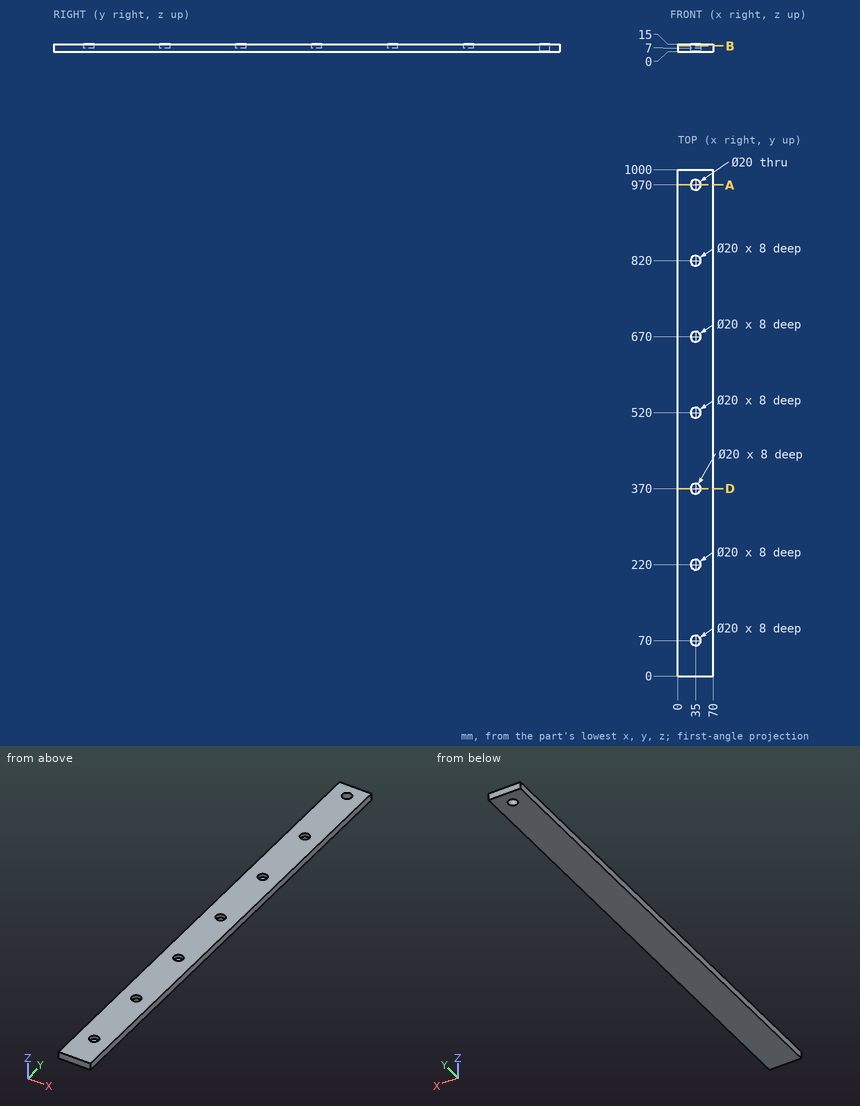
Answer from the drawing. Dimensions are ordinates in mm from the lowest x, y and z of the part. Coordinates: 2 decimals unless noted, no trailing zeros. Loops run counter-clockwise (first coordinate to the right, second up) from the corner with the lowest first, then second, coordinate; pieces in that order, holes last.
1) Consider probe 1 along X at (y, z) = (520, 9.75); probe 2 along Y at (x, z) = (27.5, 5); probe 3 along Y at (x, z) = (43, 4.75). Determine where each line is inside the solid, lowest interval first.
Results:
probe 1: x = 0 to 25, 45 to 70
probe 2: y = 0 to 963.39, 976.61 to 1000
probe 3: y = 0 to 964, 976 to 1000
2) Section A-A (y = 970) is taken. Give the vertices of the cut face in (x, z), plus the area to 3 significant figures.
Results:
outline: (0, 0) - (25, 0) - (25, 15) - (0, 15) - close; (45, 0) - (70, 0) - (70, 15) - (45, 15) - close
area: 750 mm2
3) Flat-ended cylindrical pins translate along their axes: pin 1 (12 mm diameter, centred on x = 35, y = 220, fed in from -Z); pin 2 (10 mm diameter, centred on x = 37, y = 70, fed in from +Z); pin 3 (18 mm diameter, centred on x = 35, y = 970, fed in from +Z) (3 decimals). Find the tip coordinate at first contact, or state that the pin passes through.
Results:
pin 1: stops at z = 0
pin 2: stops at z = 7
pin 3: passes through
4) Section D-D (y = 370) is taken. Give the vertices of the cut face in (x, z), plus the area to 3 significant figures.
Results:
outline: (0, 0) - (70, 0) - (70, 15) - (45, 15) - (45, 7) - (25, 7) - (25, 15) - (0, 15) - close
area: 890 mm2
5) Section B-B (z = 11.5) is taken. Give the vertices of the cut face in (x, y), plus the area to 3 significant figures.
Results:
outline: (0, 0) - (70, 0) - (70, 1000) - (0, 1000) - close; hole circle Ø20 at (35, 70); hole circle Ø20 at (35, 220); hole circle Ø20 at (35, 370); hole circle Ø20 at (35, 520); hole circle Ø20 at (35, 670); hole circle Ø20 at (35, 820); hole circle Ø20 at (35, 970)
area: 67,800 mm2
